Drawing for the job (mm, zero at the part's lowest x, y, z). Coordinates: 2 decimals unless noted, no trailing zeros. Write each loop counter-clockwise with the first axis right and the second up, starting at its lowest first coordinate (ties: lowest second). Pieces come first, ordered by that corner, then holes. Notation, with made-up numbers: (-11, -1) - (42, -1) arc R16 cw to (42, 5) - close; hole circle Ø7 at (4.5, 50.5). An arc over 180 degrees is marked (long way). Write each question's results on one line, items separated by ' | '.
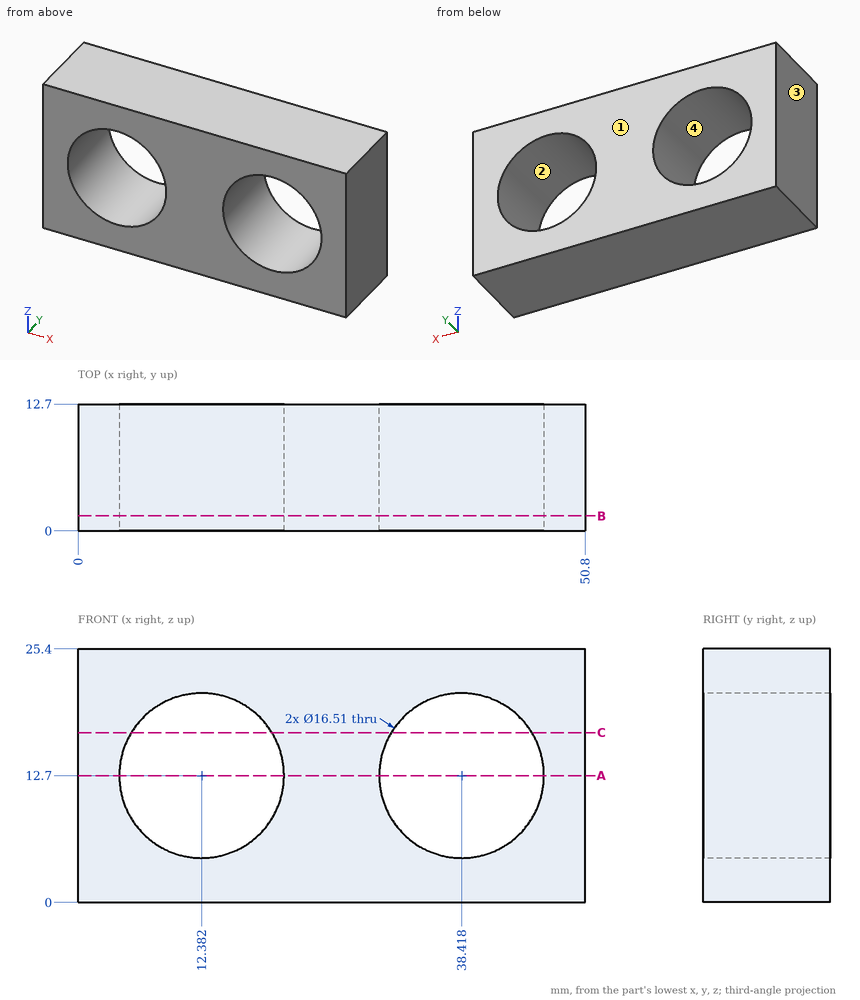
(1) Flat gauge pin, fed straight in: P1, Ø5, axis at y = 5.5, z = 12, coming from the -X side. Where does the tip first touch, or does it go through?
Return value:
P1: stops at x = 0
(2) Saw through at A-A on z = 12.7. Write the cut outline in (x, y).
Return value:
outline: (0, 0) - (4.13, 0) - (4.13, 12.7) - (0, 12.7) - close; (20.64, 0) - (30.16, 0) - (30.16, 12.7) - (20.64, 12.7) - close; (46.67, 0) - (50.8, 0) - (50.8, 12.7) - (46.67, 12.7) - close
(3) Wall check: line 1 (X direction, y = 7.5, z = 15) (1 decimal); line 2 (Z direction, x = 17.5, y = 7) (1 decimal); line 3 (Z direction, x = 45.5, y = 12) (1 decimal). Give the ranges that are in metal, low to high. Write a range as from..to.
Return value:
line 1: x = 0..4.5, 20.3..30.5, 46.3..50.8 | line 2: z = 0..6.2, 19.2..25.4 | line 3: z = 0..8.5, 16.9..25.4
(4) Two-plate mould, pull along X, no slides. Class the marked faces 1, 2, 3 and 4: released by +X, released by -X, zero draft, split by the parting line, or undercut.
Return value:
face 1: zero draft | face 2: undercut | face 3: released by -X | face 4: undercut
(5) Saw through at B-B on y = 1.5. Write the cut outline in (x, z) (1 decimal), then the cut area to 3 significant figures.
Return value:
outline: (0, 0) - (50.8, 0) - (50.8, 25.4) - (0, 25.4) - close; hole circle Ø16.5 at (12.4, 12.7); hole circle Ø16.5 at (38.4, 12.7) | area: 862 mm^2
(6) Saw through at C-C on z = 17. Write the cut outline in (x, y) (1 decimal), then the cut area to 3 significant figures.
Return value:
outline: (0, 0) - (5.3, 0) - (5.3, 12.7) - (0, 12.7) - close; (19.4, 0) - (31.4, 0) - (31.4, 12.7) - (19.4, 12.7) - close; (45.5, 0) - (50.8, 0) - (50.8, 12.7) - (45.5, 12.7) - close | area: 287 mm^2
